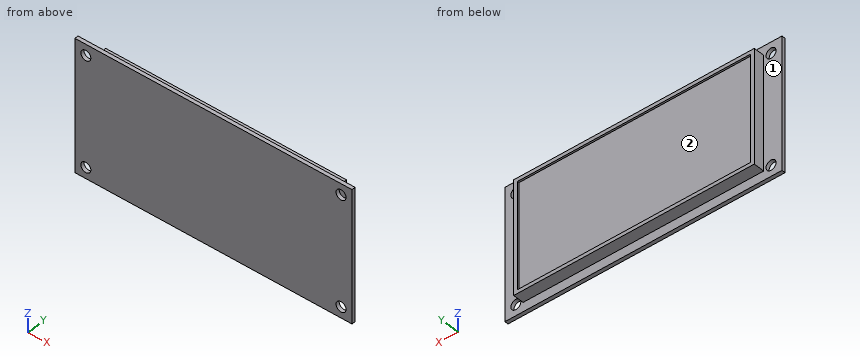
```python
from build123d import *

# Parameters (mm, degrees)
SKETCH1_W           = 76
SKETCH1_H           = 36
BOSS_EXTRUDE1_DEPTH = 1
SKETCH2_W           = 66
SKETCH2_H           = 31
BOSS_EXTRUDE2_DEPTH = 3
SKETCH3_W           = 64
SKETCH3_H           = 29
CUT_EXTRUDE1_DEPTH  = 0.5
SKETCH4_R           = 1.375
CUT_EXTRUDE2_DEPTH  = 5


with BuildPart() as part:
    # Sketch1 → Boss-Extrude1 (new body)
    with BuildSketch(Plane(origin=(0, 0, 0), x_dir=(1, 0, 0), z_dir=(0, 1, 0))):
        Rectangle(SKETCH1_W, SKETCH1_H)
    extrude(amount=BOSS_EXTRUDE1_DEPTH)

    # Sketch2 → Boss-Extrude2 (add)
    with BuildSketch(Plane(origin=(0, 1, 0), x_dir=(1, 0, 0), z_dir=(0, 1, 0))):
        Rectangle(SKETCH2_W, SKETCH2_H)
    extrude(amount=BOSS_EXTRUDE2_DEPTH)

    # Sketch3 → Cut-Extrude1 (cut)
    with BuildSketch(Plane(origin=(0, 4, 0), x_dir=(1, 0, 0), z_dir=(0, 1, 0))):
        Rectangle(SKETCH3_W, SKETCH3_H)
    extrude(amount=-CUT_EXTRUDE1_DEPTH, mode=Mode.SUBTRACT)

    # Sketch4 → Cut-Extrude2 (cut)
    with BuildSketch(Plane(origin=(0, 1, 0), x_dir=(1, 0, 0), z_dir=(0, 1, 0))):
        with Locations(Location((-35, 15, 0), (0, 0, 270))):
            Circle(SKETCH4_R)
        with Locations(Location((-35, -15, 0), (0, 0, 270))):
            Circle(SKETCH4_R)
        with Locations(Location((35, -15, 0), (0, 0, 270))):
            Circle(SKETCH4_R)
        with Locations(Location((35, 15, 0), (0, 0, 270))):
            Circle(SKETCH4_R)
    extrude(amount=-CUT_EXTRUDE2_DEPTH, mode=Mode.SUBTRACT)


solid = part.part
```
Work out the finished part from the listing and answer in its coordinate system (mm). Face numbers are marked on the shaded views. Give positions to 0.01 mm unless a question says otherwise; leave off trailing zeros. Order: outer loops, then holes, each group sorted by start corner. A loop starts at its lowest first (then second) coordinate and runs counter-clockwise, first axis right, second up. Notation, with made-up numbers: (-30.5, 51.25) -> (14.5, 51.25) arc R17 cw to (14.5, 58.25) -> close; hole circle Ø7 at (-28.75, 18.25). An arc over 180 degrees is marked (long way). Answer as CSV lines item,"result". Start each with the question number.
(1) Section C-C, the plane x = 2 is taken. Write down the section's boundary in (y, z).
(2) Each of these flat-tipped pins is pushed along its axis until it touches: pin 1 Ø4.5 at (x, z) = (-35, -15) entering from -Y; pin 2 Ø1 at (x, y) = (-2.5, 3) entering from -Z; pin 3 Ø1 at (x, y) = (22.5, 3.5) entering from +Z; pin 4 Ø1.5 at (y, z) = (2, 0) entering from +X. Where does it stop, or does it pass through?
(3) Consider line 1 along X through (y, z) = (0.5, -15) (3 decimals); line 2 along X through (y, z) = (0.65, 15.5); line 3 along Y through (x, z) = (-28, 8). Determine where each line is inside the solid, lowest interval first.
(4) Section B-B, the plane z = 7.5 is taken. Write down the section's boundary in (x, y).
(5) For a pull along Z with two mould halves and no side action, classify the marked faces 1 and 2 as released by +Z, released by -Z, zero draft, split by the parting line, or undercut.
(6) Section A-A, the plane x = 35 is taken. Write down the section's boundary in (y, z) (3 decimals).
(7) Section D-D, the plane y = 2.8 is taken. Write down the section's boundary in (x, z).
Entries:
1,outline,"(0, -18) -> (1, -18) -> (1, -15.5) -> (4, -15.5) -> (4, -14.5) -> (3.5, -14.5) -> (3.5, 14.5) -> (4, 14.5) -> (4, 15.5) -> (1, 15.5) -> (1, 18) -> (0, 18) -> close"
2,pin 1,"y = 0"
2,pin 2,"z = -15.5"
2,pin 3,"z = 15.5"
2,pin 4,"x = 33"
3,line 1,"-38 to -36.375, -33.625 to 33.625, 36.375 to 38"
3,line 2,"-38 to -36.28, -33.72 to 33.72, 36.28 to 38"
3,line 3,"0 to 3.5"
4,outline,"(-38, 0) -> (38, 0) -> (38, 1) -> (33, 1) -> (33, 4) -> (32, 4) -> (32, 3.5) -> (-32, 3.5) -> (-32, 4) -> (-33, 4) -> (-33, 1) -> (-38, 1) -> close"
5,face 1,"zero draft"
5,face 2,"undercut"
6,outline,"(0, -18) -> (1, -18) -> (1, -16.375) -> (0, -16.375) -> close; (0, -13.625) -> (1, -13.625) -> (1, 13.625) -> (0, 13.625) -> close; (0, 16.375) -> (1, 16.375) -> (1, 18) -> (0, 18) -> close"
7,outline,"(-33, -15.5) -> (33, -15.5) -> (33, 15.5) -> (-33, 15.5) -> close"
